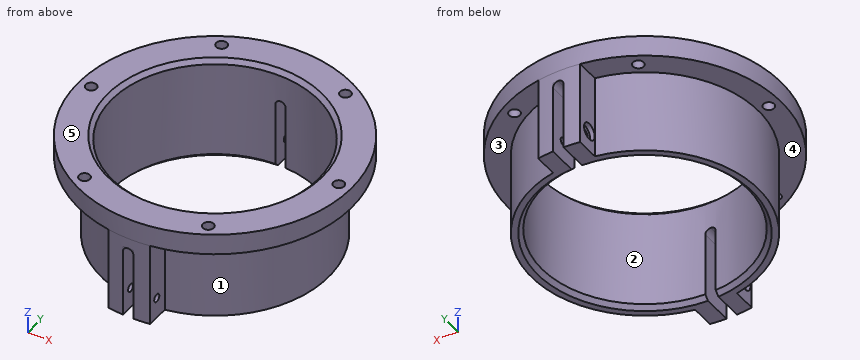
```python
from build123d import *
from build123d.topology import SkipClean

# Parameters (mm, degrees)
BOSS_EXTRUDE1_DEPTH        = 40
SKETCH3_W                  = 5
SKETCH3_H                  = 136
CUT_EXTRUDE1_DEPTH         = 35
FILLET1_R                  = 2.5
CHAMFER1_SIZE              = 2
CHAMFER2_SIZE              = 2
F_6_0_204_DIAMETER_HOLE1_D = 5.1816
CIRPATTERN1_COUNT          = 6
LPATTERN1_COUNT            = 2
LPATTERN1_PITCH            = 116.5


with BuildPart() as part:
    # Sketch1 → Revolve1 (revolve)
    with BuildSketch(Plane(origin=(0, 0, 0), x_dir=(0, 0, -1), z_dir=(1, 0, 0)), mode=Mode.PRIVATE) as revolve1_sk:
        Polygon((5, 49.1), (55, 49.1), (55, 54.1), (15, 54.1), (15, 65), (5, 65), align=None)
    revolve(revolve1_sk.sketch.rotate(Axis((0, 0, 0), (0, 0, -1)), 90), axis=Axis((0, 0, 0), (0, 0, -1)))

    # Sketch2 → Boss-Extrude1 (add)
    with BuildSketch(Plane(origin=(0, 0, -15), x_dir=(-1, 0, 0), z_dir=(0, 0, -1))):
        with BuildLine():
            Line((-10, 64.226162893), (-10, 53.167753385))
            ThreePointArc((-10, 53.167753385), (0, 54.1), (10, 53.167753385))
            Line((10, 53.167753385), (10, 64.226162893))
            ThreePointArc((10, 64.226162893), (0, 65), (-10, 64.226162893))
        make_face()
    boss_extrude1 = extrude(amount=BOSS_EXTRUDE1_DEPTH)

    # Mirror1: Boss-Extrude1 across plane
    with SkipClean():  # the faces are left unmerged after this step: merging them gives an invalid solid
        add(boss_extrude1.mirror(Plane.ZX))

    # Sketch3 → Cut-Extrude1 (cut)
    with BuildSketch(Plane(origin=(0, 0, -55), x_dir=(-1, 0, 0), z_dir=(0, 0, -1))):
        with Locations((0, -0.177278441)):
            Rectangle(SKETCH3_W, SKETCH3_H)
    extrude(amount=-CUT_EXTRUDE1_DEPTH, mode=Mode.SUBTRACT)

    # Fillet1
    # the kernel refuses this fillet: 2.5 mm, written as the material it adds along each edge
    with BuildSketch(Plane(origin=(2.5, -71.201905284, -20), x_dir=(-1, 0, 0), z_dir=(0, 1, 0))) as fillet1_piece_1_section:
        with BuildLine():
            CenterArc((FILLET1_R, -FILLET1_R), FILLET1_R, 90, 90)
            Line((0, -FILLET1_R), (0, 0))
            Line((0, 0), (FILLET1_R, 0))
        make_face()
    fillet1_piece_1 = extrude(amount=28.415592209, mode=Mode.PRIVATE)
    fillet1_piece_1 = fillet1_piece_1 - Plane(origin=(0, 0, -20.566080782), x_dir=(1, 0, 0), z_dir=(0, 0, -1)) * Cylinder(49.1, 67, mode=Mode.PRIVATE)
    fillet1_piece_1 = fillet1_piece_1 & Plane(origin=(0, 0, -20.566080782), x_dir=(-0.15384615384615422, -0.9880948137434714, 0), z_dir=(0, 0, 1)) * Cylinder(65, 67, mode=Mode.PRIVATE)
    with BuildSketch(Plane(origin=(2.5, 42.786313075, -20), x_dir=(0, 0, -1), z_dir=(0, 1, 0))) as fillet1_piece_2_section:
        with BuildLine():
            CenterArc((FILLET1_R, FILLET1_R), FILLET1_R, 180, 90)
            Line((0, FILLET1_R), (0, 0))
            Line((0, 0), (FILLET1_R, 0))
        make_face()
    fillet1_piece_2 = extrude(amount=28.415592209, mode=Mode.PRIVATE)
    fillet1_piece_2 = fillet1_piece_2 - Plane(origin=(0, 0, -20.566075474), x_dir=(1, 0, 0), z_dir=(0, 0, -1)) * Cylinder(49.1, 67, mode=Mode.PRIVATE)
    fillet1_piece_2 = fillet1_piece_2 & Plane(origin=(0, 0, -20.566075474), x_dir=(1, 0, 0), z_dir=(0, 0, 1)) * Cylinder(65, 67, mode=Mode.PRIVATE)
    with BuildSketch(Plane(origin=(-2.5, -42.786313075, -20), x_dir=(0, 0, -1), z_dir=(0, -1, 0))) as fillet1_piece_3_section:
        with BuildLine():
            CenterArc((FILLET1_R, FILLET1_R), FILLET1_R, 180, 90)
            Line((0, FILLET1_R), (0, 0))
            Line((0, 0), (FILLET1_R, 0))
        make_face()
    fillet1_piece_3 = extrude(amount=28.415592209, mode=Mode.PRIVATE)
    fillet1_piece_3 = fillet1_piece_3 - Plane(origin=(0, 0, -20.566082494), x_dir=(1, 0, 0), z_dir=(0, 0, -1)) * Cylinder(49.1, 67, mode=Mode.PRIVATE)
    fillet1_piece_3 = fillet1_piece_3 & Plane(origin=(0, 0, -20.566082494), x_dir=(-0.15384615384615422, -0.9880948137434714, 0), z_dir=(0, 0, 1)) * Cylinder(65, 67, mode=Mode.PRIVATE)
    with BuildSketch(Plane(origin=(-2.5, 71.201905284, -20), x_dir=(1, 0, 0), z_dir=(0, -1, 0))) as fillet1_piece_4_section:
        with BuildLine():
            CenterArc((FILLET1_R, -FILLET1_R), FILLET1_R, 90, 90)
            Line((0, -FILLET1_R), (0, 0))
            Line((0, 0), (FILLET1_R, 0))
        make_face()
    fillet1_piece_4 = extrude(amount=28.415592209, mode=Mode.PRIVATE)
    fillet1_piece_4 = fillet1_piece_4 - Plane(origin=(0, 0, -20.566085883), x_dir=(1, 0, 0), z_dir=(0, 0, -1)) * Cylinder(49.1, 67, mode=Mode.PRIVATE)
    fillet1_piece_4 = fillet1_piece_4 & Plane(origin=(0, 0, -20.566085883), x_dir=(1, 0, 0), z_dir=(0, 0, 1)) * Cylinder(65, 67, mode=Mode.PRIVATE)
    add([fillet1_piece_1, fillet1_piece_2, fillet1_piece_3, fillet1_piece_4])

    # Chamfer1
    chamfer1_edges = [part.edges().sort_by_distance(p)[0] for p in [
        (-49.1, 0, -55),
        (35.591853, -33.823512532, -55),
    ]]
    chamfer(chamfer1_edges, length=CHAMFER1_SIZE)

    # Chamfer2
    chamfer2_edges = [part.edges().sort_by_distance(p)[0] for p in [
        (-49.1, 0, -5),
    ]]
    chamfer(chamfer2_edges, length=CHAMFER2_SIZE)

    # #6 (0.204) Diameter Hole1 (through all)
    with Locations(Plane.XY.offset(-5)):
        with Locations((-29.625, 51.312005174)):
            f_6_0_204_diameter_hole1 = Hole(F_6_0_204_DIAMETER_HOLE1_D / 2)

    # CirPattern1: #6 (0.204) Diameter Hole1 ×6 about axis
    with SkipClean():  # the faces are left unmerged after this step: merging them gives an invalid solid
        cirpattern1_axis = Axis((0, 0, 0), (0, 0, 1))
        for i in range(1, CIRPATTERN1_COUNT):
            add(f_6_0_204_diameter_hole1.rotate(cirpattern1_axis, i * 360 / CIRPATTERN1_COUNT), mode=Mode.SUBTRACT)

    # Sketch8 → CBORE for #6 Binding Head Machine Screw1 (revolve, cut)
    with SkipClean():  # the faces are left unmerged after this step: merging them gives an invalid solid
        with BuildSketch(Plane(origin=(-10, -59.226162893, -45), x_dir=(0, 0, 1), z_dir=(0, 1, 0))):
            Polygon((0, 0), (0, 26.140824014), (1.89865, 25), (1.89865, 2.2098), (3.96875, 2.2098), (3.96875, 0), align=None)
        cbore_for_6_binding_head_machine_screw1 = revolve(axis=Axis((-16.35, -59.226162893, -45), (1, 0, 0)), mode=Mode.SUBTRACT)

    # LPattern1: CBORE for #6 Binding Head Machine Screw1 ×2
    with SkipClean():  # the faces are left unmerged after this step: merging them gives an invalid solid
        with Locations(*[(0, i * LPATTERN1_PITCH, 0) for i in range(1, LPATTERN1_COUNT)]):
            add(cbore_for_6_binding_head_machine_screw1, mode=Mode.SUBTRACT)


solid = part.part
```
Here's how the part is built. I have some questions about the finished solid (model axes, mm). Face numbers are marked on the shaded views. A direction names the side the tool comes from. Give positions to 0.01 mm unless a question says otherwise; leave off trailing zeros. Loops run counter-clockwise (first coordinate to the right, second up) from the corner with the lowest first, then second, coordinate; pieces in that order, holes last. Notation, with made-up numbers: (65, -4.5) -> (113, -4.5) arc R26 ccw to (113, 12.5) -> close; hole circle Ø6 at (24.5, -24). An arc over 180 degrees is marked (long way). Use one line per item in the form item = value. Start each with the question number.
1) Please list where these lines run through material, in increasing order: line 1 along X through (y, z) = (-1.5, -26); line 2 along Y through (x, z) = (-8.6, -45); line 3 along Z through (x, y) = (-26, 52).
2) Which directions (+Z, -Z, +X, -X, +Y, -Y) give clear straight access to the entire face, cutting with the end or side of a thin tool? Please do the marked faces 4 and 5.
3) Imagine slicing it at C-C (z = -12). Please give me the cut outline in (x, y) (3 decimals), then the cut area to 3 significant figures.
4) For P1, Ø5, axis at x = -1, z = -26.5, coming from the +Y side; P2, Ø6.5, axis at x = -29.62, y = -51.31, coming from the -Z side; P3, Ø5.5, axis at y = -56.5, z = -30.5, coming from the -X side, each with a flat end and sliding along its axis, tell me the tip position at first contact or that it passes through.
5) Imagine slicing it at A-A (y = 0). Please give me the cut outline in (x, z), then the cut area to 3 significant figures.
6) Imagine slicing it at B-B (z = -25). Please give me the cut outline in (x, y).
7) Thinking about a two-plate mould opening in Y: for the marked faces 1, 2 and 3, which applies, +Y half, -Y half, draft (parallel to the pull), parting line (faces both ways), or undercut?
8) Imagine slicing it at D-D (x = -5). Count the separate pieces of the cut face and the enclosed holes in it, then the cut area to 3 significant figures.
Check values:
q1.line_1 = -54.08 to -49.08, 49.08 to 54.08
q1.line_2 = -64.43 to -63.19, -55.26 to -48.34, 48.34 to 53.31, 61.24 to 64.43
q1.line_3 = -15 to -5
q2.face_4 = -Z, -X
q2.face_5 = +Z, +X, -X, +Y, -Y
q3.outline = circle Ø130 at (0, 0); hole circle Ø5.182 at (-59.25, 0); hole circle Ø98.2 at (0, 0); hole circle Ø5.182 at (-29.625, -51.312); hole circle Ø5.182 at (-29.625, 51.312); hole circle Ø5.182 at (29.625, -51.312); hole circle Ø5.182 at (29.625, 51.312); hole circle Ø5.182 at (59.25, 0)
q3.area = 5,570 mm^2
q4.P1 = 64.95
q4.P2 = -15
q4.P3 = -10
q5.outline = (-65, -15) -> (-61.84, -15) -> (-61.84, -5) -> (-65, -5) -> close; (-56.66, -15) -> (-54.1, -15) -> (-54.1, -55) -> (-51.1, -55) -> (-49.1, -53) -> (-49.1, -7) -> (-51.1, -5) -> (-56.66, -5) -> close; (49.1, -53) -> (51.1, -55) -> (54.1, -55) -> (54.1, -15) -> (56.66, -15) -> (56.66, -5) -> (51.1, -5) -> (49.1, -7) -> close; (61.84, -15) -> (65, -15) -> (65, -5) -> (61.84, -5) -> close
q5.area = 606 mm^2
q6.outline = (-10, -64.23) arc R65 ccw to (-2.5, -64.95) -> (-2.5, -49.04) arc R49.1 cw to (-2.5, 49.04) -> (-2.5, 64.95) arc R65 ccw to (-10, 64.23) -> (-10, 53.17) arc R54.1 ccw to (-10, -53.17) -> close; (2.5, -64.95) arc R65 ccw to (10, -64.23) -> (10, -53.17) arc R54.1 ccw to (10, 53.17) -> (10, 64.23) arc R65 ccw to (2.5, 64.95) -> (2.5, 49.04) arc R49.1 cw to (2.5, -49.04) -> close
q7.face_1 = parting line
q7.face_2 = undercut
q7.face_3 = draft
q8.separate_pieces = 2
q8.enclosed_holes = 2
q8.area = 1,570 mm^2
